Here's how the part is built. I have some questions about the finished solid (model axes, mm). Face numbers are marked on the shaded views. A direction names the side the tool comes from. Coordinates: 2 decimals unless noted, no trailing zeros. Order: outer loops, then holes, each group sorted by start corner. A loop starts at its lowest first (then second) coordinate and runs counter-clockwise, first axis right, second up.
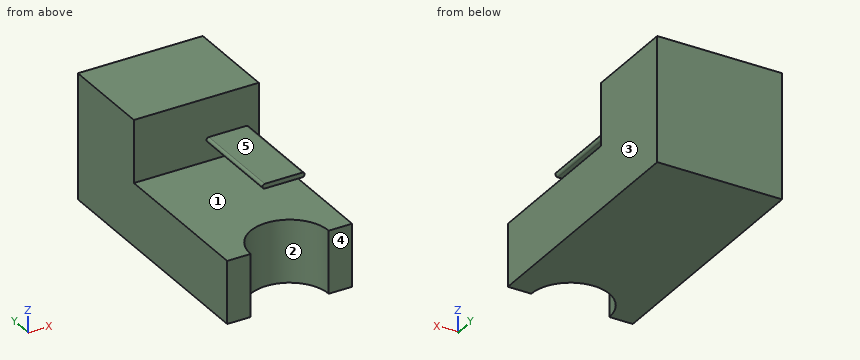
Autodesk Inventor part; units mm, degrees
ref_plane "YZ Plane" through (0, 0, 0) normal (1, 0, 0) x (0, 1, 0)
ref_plane "XZ Plane" through (0, 0, 0) normal (0, 1, 0) x (-1, 0, 0)
ref_plane "XY Plane" through (0, 0, 0) normal (0, 0, 1) x (1, 0, 0)
sketch "Sketch4" plane through (0, 0, 0) normal (1, 0, 0) x (0, 1, 0)
  line L0 (0, 0) -> (-101.6, 0)
  line L1 (-101.6, 0) -> (-101.6, -50.8)
  line L2 (-101.6, -50.8) -> (0, -50.8)
  line L3 (0, -50.8) -> (0, 0)
  dimension "d6" = 101.6
  dimension "d7" = 50.8
extrude "Extrusion3" add sketch "Sketch4" along normal blind 50.8
sketch "Sketch5" plane through (0, -101.6, 0) normal (0, 0, 1) x (1, 0, 0)
  line L0 (0, 0) -> (50.8, 0)
  arc A0 (41.275, 0) -> (9.525, 0) centre (25.4, 0) ccw
  line L1 (0, 101.6) -> (0, 0)
  dimension "d10" = 15.875
  dimension "d11" = 31.75
  dimension "d12" = 50.8
  dimension "d13" = 9.525
extrude "Extrusion4" cut sketch "Sketch5" against normal through all
sketch "Sketch6" plane through (0, -101.6, -50.8) normal (0, -1, 0) x (1, 0, 0)
  line L0 (0, 50.8) -> (9.525, 50.8)
  line L1 (50.8, 50.8) -> (50.8, 0)
  line L2 (0, 50.8) -> (50.8, 50.8)
  line L3 (50.8, 50.8) -> (50.8, 25.4)
  line L4 (50.8, 25.4) -> (0, 25.4)
  line L5 (0, 25.4) -> (0, 50.8)
extrude "Extrusion5" cut sketch "Sketch6" against normal blind 63.5
sketch "Sketch7" plane through (0, -38.1, -50.8) normal (0, -1, 0) x (1, 0, 0)
  line L0 (46.6725, 33.9725) -> (29.5275, 33.9725) construction
  line L1 (45.72, 34.925) -> (30.48, 34.925)
  line L2 (30.48, 33.02) -> (45.72, 33.02)
  arc A0 (45.72, 33.02) -> (45.72, 34.925) centre (45.72, 33.9725) ccw
  arc A1 (30.48, 34.925) -> (30.48, 33.02) centre (30.48, 33.9725) ccw
  line L3 (0, 50.8) -> (50.8, 50.8)
  line L4 (50.8, 50.8) -> (50.8, 25.4)
  line L5 (41.275, 25.4) -> (9.525, 25.4)
  point P0 (38.1, 33.9725)
  dimension "d18" = 17.145
  dimension "d19" = 1.905
  dimension "d20" = 50.8
  dimension "d21" = 4.1275
  dimension "d22" = 7.62
extrude "Extrusion6" add sketch "Sketch7" along normal blind 38.1
equation "\"d13\" = -0.5 * d11 + 0.5 * d12"
properties part number "graber base"
Q1. We'd pull the mould along X, two halves only. Please class the marked faces 1, 2 and 3: pulls with the +X half, pulls with the -X half, needs draft (parallel to the pull), parting line crosses it, or undercut.
Q2. If we section it at B-B on x = 42.5: Write out the boundary of the cut face in (y, z) (3 decimals).
Q3. If we section it at C-C on z = -38: Write out the boundary of the cut face in (x, y) (3 decimals).
Q4. If we section it at A-A on y = -46: Write out the boundary of the cut face in (x, z) (1 decimal), then the cut area to 3 significant figures.
Q5. I need wall thicknesses on L1, parallel to Z at x = 22.5, y = -66; L2, parallel to Y at x = 26, z = -32; L3, parallel to Y at x = 35.5, z = -12.5. Which ranges of each line are inside material? Lowest first, please.
Q6. For the marked faces 4 and 5, which set-ups out of +Z, -Z, +X, -X, +Y, -Y let a thin tool reach every point of the face, with its end or its side?
Q7. Will these pins go through, and if not, where does the flat tip stop? pin 1 (12.5 mm diameter, centred on x = 37, z = -8.5, fed in from -Y); pin 2 (1 mm diameter, centred on x = 40.5, z = -16.5, fed in from -Y); pin 3 (4.5 mm diameter, centred on x = 39, y = -63.5, fed in from +Z) (3 decimals); pin 4 (1.5 mm diameter, centred on x = 16, z = -32, fed in from +Y).
Q8. If we section it at D-D on y = -83: Write out the boundary of the cut face in (x, z), then the cut area to 3 significant figures.
Reply:
1. face 1: needs draft
1. face 2: undercut
1. face 3: pulls with the +X half
2. outline: (-101.6, -50.8) - (0, -50.8) - (0, 0) - (-38.1, 0) - (-38.1, -15.875) - (-76.2, -15.875) - (-76.2, -17.78) - (-38.1, -17.78) - (-38.1, -25.4) - (-101.6, -25.4) - close
3. outline: (0, -101.6) - (9.525, -101.6) arc R15.875 cw to (41.275, -101.6) - (50.8, -101.6) - (50.8, 0) - (0, 0) - close
4. outline: (0, -50.8) - (50.8, -50.8) - (50.8, -25.4) - (0, -25.4) - close; (30.5, -17.8) - (45.7, -17.8) arc R1 ccw to (45.7, -15.9) - (30.5, -15.9) arc R1 ccw to start
4. area: 1,320 mm2
5. L1: z = -50.8 to -25.4
5. L2: y = -85.74 to 0
5. L3: y = -38.1 to 0
6. face 4: +Z, -Z, +X, -X, -Y
6. face 5: +Z, +X, -X, -Y
7. pin 1: stops at y = -38.1
7. pin 2: stops at y = -76.2
7. pin 3: stops at z = -15.875
7. pin 4: stops at y = 0
8. outline: (0, -50.8) - (50.8, -50.8) - (50.8, -25.4) - (0, -25.4) - close
8. area: 1,290 mm2
